Input: dimensioned drawing with shaded views. Units: mm. Origin: part minimum x, y, z. Round coordinates to 2 decimals unless told otherwise and drop trailing zeros. Loops run counter-clockwise (first coordinate to the right, second up) from the corner with the lowest first, then second, coordinate; pieces in that order, holes last. Notation, with made-up numbers: (62, -1) - (111, -1) arc R21 ccw to (111, 16) - close; hole circle Ø1 at (82, 7.5). An arc over 180 degrees is marked (long way). Answer as CSV lines item,"result".
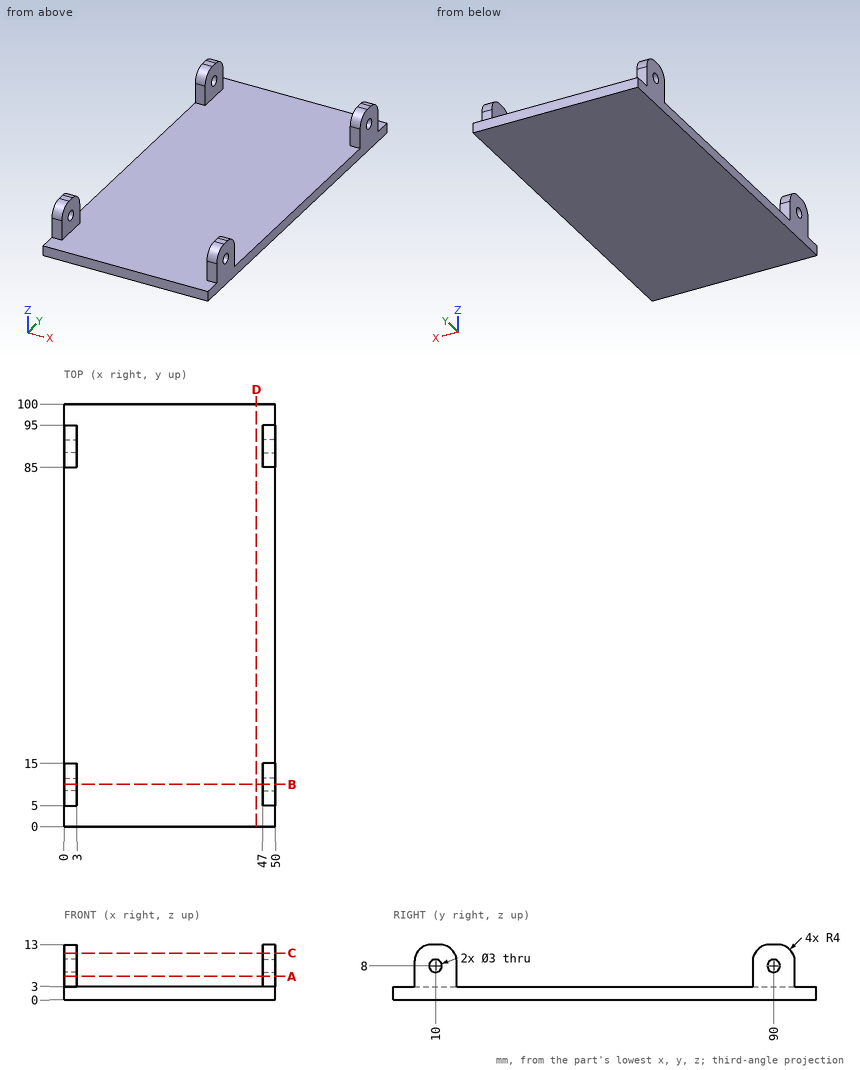
(1) Material intervals for line 1 along Z through (x, y) = (48.4, 10); line 2 along X through (y, z) = (11.5, 3.5); line 3 along Z through (x, y) = (6, 65), sorted ascending.
Findings below:
line 1,"0 to 6.5, 9.5 to 13"
line 2,"0 to 3, 47 to 50"
line 3,"0 to 3"
(2) Section B-B (y = 10). Output: boundary loops of the cut face in (x, z).
Findings below:
outline,"(0, 0) - (50, 0) - (50, 6.5) - (47, 6.5) - (47, 3) - (3, 3) - (3, 6.5) - (0, 6.5) - close; (0, 9.5) - (3, 9.5) - (3, 13) - (0, 13) - close; (47, 9.5) - (50, 9.5) - (50, 13) - (47, 13) - close"
(3) Pin query (flat end, axial travel): P1, Ø3.5, axis at x = 48.5, z = 5.5, coming from the +Y side; P2, Ø1.5, axis at x = 1.5, z = 4.5, coming from the -Y side; P3, Ø2.5, axis at y = 90, z = 8, coming from the +X side. Return the tip coordinate at first contact, or that it passes through.
Findings below:
P1,"y = 95"
P2,"y = 5"
P3,"through"
(4) Section A-A (z = 5.5). Output: boundary loops of the cut face in (x, y).
Findings below:
outline,"(0, 5) - (3, 5) - (3, 15) - (0, 15) - close; (0, 85) - (3, 85) - (3, 95) - (0, 95) - close; (47, 5) - (50, 5) - (50, 15) - (47, 15) - close; (47, 85) - (50, 85) - (50, 95) - (47, 95) - close"
(5) Section C-C (z = 11). Output: boundary loops of the cut face in (x, y).
Findings below:
outline,"(0, 5.54) - (3, 5.54) - (3, 14.46) - (0, 14.46) - close; (0, 85.54) - (3, 85.54) - (3, 94.46) - (0, 94.46) - close; (47, 5.54) - (50, 5.54) - (50, 14.46) - (47, 14.46) - close; (47, 85.54) - (50, 85.54) - (50, 94.46) - (47, 94.46) - close"
(6) Section D-D (x = 45.5). Output: boundary loops of the cut face in (y, z), and give its area (3 significant figures).
Findings below:
outline,"(0, 0) - (100, 0) - (100, 3) - (0, 3) - close"
area,"300 mm2"
